Input: part model. Units: mm. Frame: model coordinates. Face numbers are marked on the shaded views. A direction names the side the tool comes from. Round coordinates to 2 decimals unless told otherwise and drop trailing zeros. Loops run counter-clockwise (first coordinate to the right, second up) from the corner with the lowest first, then second, coordinate; pieces in that order, holes last. Notation, with made-up numbers: (-37, 60.5) - (-17, 60.5) arc R17 ccw to (-17, 66.5) - close; hole circle Ø11 at (25, 3.25). An arc over 180 degrees is marked (long way). Use CSV: the item, a comma, the result in double quotes. Start each with the question number.
1. Cut plane D-D (z = 6.75). Return loops of the section in (x, y).
2. Cut plane C-C (y = -1.25). Return loops of the section in (x, z).
3. Cut plane B-B (x = -2.25). Return loops of the section in (y, z).
4. Access query for the marked faces 4 and 5. Directions: +Z, -Z, +X, -X, +Y, -Y. A direction counts if a zero-diameter tool reaches every point of the face in a straight line with its end or side. Return the directions, or none.
5. Pin query (flat end, axial travel): P1, Ø1.4, axis at y = -2.5, z = 7, coming from the +X side; P2, Ø2, axis at x = -2.5, y = -1.5, coming from the -Z side; P3, Ø3.5, axis at x = 2.5, z = 5.5, coming from the -Y side; P4, Ø6, axis at x = 0.5, z = 3, coming from the +Y side. Return the tip coordinate at first contact, or that it passes through.
6. Material intervals for probe 1 along Z at (x, y) = (0, -2.5); probe 2 along Y at (x, z) = (4.75, 3.75); probe 3 along X at (y, z) = (-0.25, -1), sorted ascending. Write a range as from..to.
7. Cut plane A-A (z = -1.5). Return loops of the section in (x, y), and give its area (3 significant figures).
8. Pull-direction query (Z, two-part tool) for the marked faces 1, 2 and 3; classes: +Z half, -Z half, draft (parallel to the pull), parting line (faces both ways), or undercut.
```python
from build123d import *

# Parameters (mm, degrees)
F1_DEPTH = 1.5
F3_DEPTH = 1.3
F5_DEPTH = 3.9
F6_R     = 3
F7_DEPTH = 6.701
F9_DEPTH = 25


with BuildPart() as f1:
    # F0 (on Front) → F1 (new body)
    with BuildSketch(Plane.XZ):
        with BuildLine():
            Line((-5.7, 10.7), (-5.7, 0))
            ThreePointArc((-5.7, 0), (-4.030509, -4.030509), (0, -5.7))
            ThreePointArc((0, -5.7), (4.030509, -4.030509), (5.7, 0))
            Line((5.7, 0), (5.7, 10.7))
            Line((5.7, 10.7), (-5.7, 10.7))
        make_face()
    extrude(amount=F1_DEPTH)

    # F2 (on face) → F3 (join)
    with BuildSketch(Plane.XZ.offset(1.5)):
        with BuildLine():
            Line((4.25, 0), (4.25, 9.25))
            Line((4.25, 9.25), (-4.25, 9.25))
            Line((-4.25, 9.25), (-4.25, 0))
            ThreePointArc((-4.25, 0), (0, -4.25), (4.25, 0))
        make_face()
    extrude(amount=F3_DEPTH)

    # F4 (on face) → F5 (join)
    with BuildSketch(Plane.XZ.offset(2.8)):
        with BuildLine():
            ThreePointArc((3.15, 0), (0, 3.15), (-3.15, 0))
            ThreePointArc((-3.15, 0), (0, -3.15), (3.15, 0))
        make_face()
    extrude(amount=F5_DEPTH)

    # F6 (on face) → F7 (cut, through all)
    with BuildSketch(Plane.XZ.offset(6.7)):
        Circle(F6_R)
    extrude(amount=-F7_DEPTH, mode=Mode.SUBTRACT)

    # F8 (on face) → F9 (cut)
    with BuildSketch(Plane(origin=(-4.25, 0, 0), x_dir=(0, -1, 0), z_dir=(-1, 0, 0))):
        Polygon((3.389618, 4.891665), (3.389618, 2.457727), (6.718387, 0), (7.86377, 0), (7.899563, 4.891665), align=None)
    extrude(amount=-F9_DEPTH, mode=Mode.SUBTRACT)


solid = f1.part
```
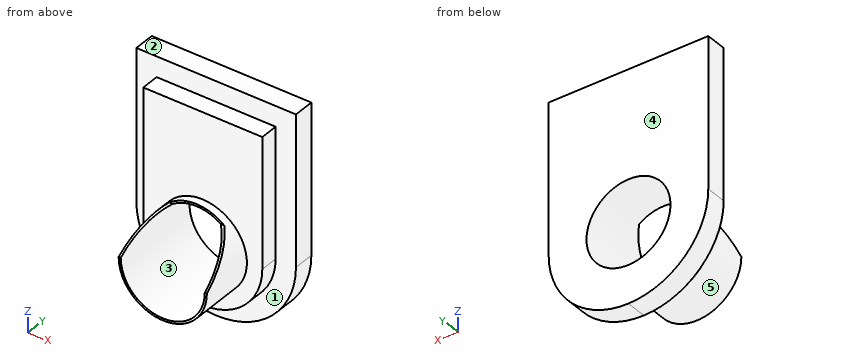
Established:
1,outline,"(-5.7, -1.5) - (-4.25, -1.5) - (-4.25, -2.8) - (4.25, -2.8) - (4.25, -1.5) - (5.7, -1.5) - (5.7, 0) - (-5.7, 0) - close"
2,outline,"(-5.7, 0) arc R5.7 ccw to (0, -5.7) arc R5.7 ccw to (5.7, 0) - (5.7, 10.7) - (-5.7, 10.7) - close; hole circle Ø6 at (0, 0)"
3,outline,"(-6.7, -2.2) - (-2.8, -2.2) - (-2.8, -3.61) - (-1.5, -3.61) - (-1.5, -5.24) - (0, -5.24) - (0, -1.98) - (-6.7, -1.98) - close; (-4.03, 1.98) - (0, 1.98) - (0, 10.7) - (-1.5, 10.7) - (-1.5, 9.25) - (-2.8, 9.25) - (-2.8, 2.2) - (-3.73, 2.2) - close"
4,face 4,"+Z, -Z, +X, -X, +Y"
4,face 5,"-Y"
5,P1,"stops at x = 4.25"
5,P2,"stops at z = -5.5"
5,P3,"stops at y = -2.8"
5,P4,"stops at y = 0"
6,probe 1,"z = -4.25..-3, 3..9.25"
6,probe 2,"y = -1.5..0"
6,probe 3,"x = -5.61..-2.83, 2.83..5.61"
7,outline,"(-5.5, -1.5) - (-3.98, -1.5) - (-3.98, -2.8) - (-2.77, -2.8) - (-2.77, -6.7) - (-2.6, -6.7) - (-2.6, 0) - (-5.5, 0) - close; (2.6, -6.7) - (2.77, -6.7) - (2.77, -2.8) - (3.98, -2.8) - (3.98, -1.5) - (5.5, -1.5) - (5.5, 0) - (2.6, 0) - close"
7,area,"13.6 mm2"
8,face 1,"draft"
8,face 2,"+Z half"
8,face 3,"undercut"
